Read the model definition and answer for the solid it produces. Units are mm, in the model's axes. A direction names the side the tool comes from. Give positions to 0.01 mm unless a question says otherwise; leave off trailing zeros. Loops run counter-clockwise (first coordinate to the right, second up) from the corner with the lowest first, then second, coordinate; pieces in that order, holes last. Notation, with made-up numbers: (70, 26.5) - (87, 26.5) arc R22 cw to (87, 65.5) - close; hole circle Ø3 at (-4.75, -29.75). An arc over 180 degrees is marked (long way). Write item = value, one per line. Start each with the question number.
from build123d import *

# Parameters (mm, degrees)
SKETCH1_W                                  = 16
SKETCH1_H                                  = 18
SKETCH1_W_2                                = 12
SKETCH1_H_2                                = 14
EXTRUDE_THIN1_DEPTH                        = 2
BOSS_EXTRUDE1_DEPTH                        = 2
SKETCH3_R                                  = 3
BOSS_EXTRUDE2_DEPTH                        = 2
BOSS_EXTRUDE2_TAPER                        = 35
SKETCH13_W                                 = 12
SKETCH13_H                                 = 1
BOSS_EXTRUDE4_DEPTH                        = 4
CUT_EXTRUDE5_REACH                         = 28.215
SKETCH11_R                                 = 0.5
MIRROR4_AT_THE_SECOND_PLANE_COPY_1_REACH   = 28.215
MIRROR4_AT_THE_SECOND_PLANE_COPY_1_SKETC_R = 0.5


with BuildPart() as part:
    # Sketch1 → Extrude-Thin1 (new, symmetric)
    with BuildSketch(Plane.XY):
        Rectangle(SKETCH1_W, SKETCH1_H)
        Rectangle(SKETCH1_W_2, SKETCH1_H_2, mode=Mode.SUBTRACT)
    extrude_thin1 = extrude(amount=EXTRUDE_THIN1_DEPTH, both=True)

    # Sketch2 → Boss-Extrude1 (add)
    with BuildSketch(Plane(origin=(8, 0, 0), x_dir=(0, 0, -1), z_dir=(1, 0, 0))):
        with BuildLine():
            Line((2, 9), (-15.5, 9))
            ThreePointArc((-15.5, 9), (-24.5, 0), (-15.5, -9))
            Line((-15.5, -9), (2, -9))
            Line((2, -9), (2, 9))
        make_face()
    boss_extrude1 = extrude(amount=-BOSS_EXTRUDE1_DEPTH)

    # Sketch3 → Boss-Extrude2 (add)
    with BuildSketch(Plane(origin=(8, 0, 0), x_dir=(0, 0, -1), z_dir=(1, 0, 0))):
        with Locations((-15.5, 0)):
            Circle(SKETCH3_R)
    boss_extrude2 = extrude(amount=BOSS_EXTRUDE2_DEPTH, taper=BOSS_EXTRUDE2_TAPER)

    # Mirror3: Extrude-Thin1, Boss-Extrude1, Boss-Extrude2 across plane
    add(extrude_thin1.mirror(Plane(origin=(0, 0, 0), x_dir=(0, 0, 1), z_dir=(1, 0, 0))))
    add(boss_extrude1.mirror(Plane(origin=(0, 0, 0), x_dir=(0, 0, 1), z_dir=(1, 0, 0))))
    add(boss_extrude2.mirror(Plane(origin=(0, 0, 0), x_dir=(0, 0, 1), z_dir=(1, 0, 0))))

    # Sketch13 → Boss-Extrude4 (add)
    with BuildSketch(Plane.XY.offset(2)):
        with Locations((0, 6.5)):
            Rectangle(SKETCH13_W, SKETCH13_H)
    boss_extrude4 = extrude(amount=-BOSS_EXTRUDE4_DEPTH)

    # Mirror5: Boss-Extrude4 across plane
    add(boss_extrude4.mirror(Plane.ZX))

    # Sketch11 → Cut-Extrude5 (cut, up to next)
    with BuildSketch(Plane.XY.offset(2), mode=Mode.PRIVATE) as cut_extrude5_sk1:
        with Locations((-4.5, 7.5)):
            Circle(SKETCH11_R)
    cut_extrude5_tool1 = extrude(cut_extrude5_sk1.sketch, amount=-CUT_EXTRUDE5_REACH, mode=Mode.PRIVATE) & part.part
    cut_extrude5 = cut_extrude5_tool1.solids().sort_by_distance((-4.5, 7.5, 2))[0]
    add(cut_extrude5, mode=Mode.SUBTRACT)

    # Mirror4: Cut-Extrude5 across plane
    add(cut_extrude5.mirror(Plane.ZX), mode=Mode.SUBTRACT)

    # Mirror4 at the second plane: Cut-Extrude5 across plane
    add(cut_extrude5.mirror(Plane(origin=(0, 0, 0), x_dir=(0, 0, 1), z_dir=(1, 0, 0))), mode=Mode.SUBTRACT)

    # Mirror4 at the second plane copy 1 sketc → Mirror4 at the second plane copy 1 (cut, up to next)
    with BuildSketch(Plane(origin=(0, 0, 2), x_dir=(-1, 0, 0), z_dir=(0, 0, 1)), mode=Mode.PRIVATE) as mirror4_at_the_second_plane_copy_1_sk1:
        with Locations((-4.5, 7.5)):
            Circle(MIRROR4_AT_THE_SECOND_PLANE_COPY_1_SKETC_R)
    mirror4_at_the_second_plane_copy_1_tool1 = extrude(mirror4_at_the_second_plane_copy_1_sk1.sketch, amount=-MIRROR4_AT_THE_SECOND_PLANE_COPY_1_REACH, mode=Mode.PRIVATE) & part.part
    add(mirror4_at_the_second_plane_copy_1_tool1.solids().sort_by_distance((4.5, -7.5, 2))[0], mode=Mode.SUBTRACT)


solid = part.part
1. Given P1, Ø6, axis at x = 5, y = -4.5, coming from the +Z side; P2, Ø6, axis at x = -0.5, y = -1.5, coming from the +Z side; P3, Ø0.9, axis at x = 0, y = 7, coming from the +Z side; P4, Ø5.5, axis at y = 0.5, z = 8, coming from the +X side, each flat-ended and moving along its own axis, determine where each tip first touches the part or whether it passes through.
2. A cutting plane is placed at D-D on y = -7.5. Give the vertices of the cut face in (x, z).
3. Consider line 1 along Y through (x, z) = (4.5, 0.9); line 2 along X through (y, z) = (-7.5, -0.4); line 3 along X through (y, z) = (-3.5, 20.75). Determine where each line is inside the solid, lowest interval first. Write a range as [from, to].
4. For a pull along Y with two mould halves and no side action, classify faces 1 (the cylindrical face through (-7.014, 0.198, 24.498)), 2 (the flat face through (0, -8, 2)), 3 (the flat face through (0, 9, 1)), 4 (the cylindrical face through (-4.608, 7.012, 0.028)) as released by +Y, released by -Y, zero draft, split by the parting line, or undercut.
5. A tool of negligible diameter and unlimited length cuts with its end or side. For faces 5 (the flat face through (0, 6, 0)), 6 (the cylindrical face through (7.014, 0.198, 24.498)), 7 (the flat face through (0, 8, 2)), from which of +Z, -Z, +X, -X, +Y, -Y can it reach the whole face along a straight path? Write none if from no direction.
6. A cutting plane is placed at A-A on z = 5. Give the vertices of the cut face in (x, y).
7. A cutting plane is placed at B-B on x = -4.5. Give the vertices of the cut face in (y, z), and give its area (3 significant figures).
8. A cutting plane is placed at C-C on z = 1.5. Give the vertices of the cut face in (x, y), and give its area (3 significant figures).
Reply:
q1.P1 = 24.34
q1.P2 = through
q1.P3 = 2
q1.P4 = 8
q2.outline = (-8, -2) - (-5, -2) - (-5, 2) - (-6, 2) - (-6, 20.47) - (-8, 20.47) - close; (-4, -2) - (4, -2) - (4, 2) - (-4, 2) - close; (5, -2) - (8, -2) - (8, 20.47) - (6, 20.47) - (6, 2) - (5, 2) - close
q3.line_1 = [-9, -8], [-7, -6], [6, 7], [8, 9]
q3.line_2 = [-8, -5], [-4, 4], [5, 8]
q3.line_3 = [-8, -6], [6, 8]
q4.face_1 = split by the parting line
q4.face_2 = zero draft
q4.face_3 = released by +Y
q4.face_4 = undercut
q5.face_5 = +Z, -Z
q5.face_6 = +Z, +X, -X
q5.face_7 = +Z, +Y, -Y
q6.outline = (-8, -9) - (-6, -9) - (-6, 9) - (-8, 9) - close; (6, -9) - (8, -9) - (8, 9) - (6, 9) - close
q7.outline = (-9, -2) - (-8, -2) - (-8, 2) - (-9, 2) - close; (-7, -2) - (-6, -2) - (-6, 2) - (-7, 2) - close; (6, -2) - (7, -2) - (7, 2) - (6, 2) - close; (8, -2) - (9, -2) - (9, 2) - (8, 2) - close
q7.area = 16.0 mm^2
q8.outline = (-8, -9) - (8, -9) - (8, 9) - (-8, 9) - close; hole (-6, -6) - (6, -6) - (6, 6) - (-6, 6) - close; hole circle Ø1 at (-4.5, -7.5); hole circle Ø1 at (-4.5, 7.5); hole circle Ø1 at (4.5, -7.5); hole circle Ø1 at (4.5, 7.5)
q8.area = 141 mm^2
